Autodesk Inventor part; units mm, degrees
ref_plane "YZ Plane" through (0, 0, 0) normal (1, 0, 0) x (0, 1, 0)
ref_plane "XZ Plane" through (0, 0, 0) normal (0, 1, 0) x (-1, 0, 0)
ref_plane "XY Plane" through (0, 0, 0) normal (0, 0, 1) x (1, 0, 0)
sketch "Sketch1" plane through (0, 0, 0) normal (0, 1, 0) x (-1, 0, 0)
  circle A0 centre (0, 0) radius 100
  dimension "d0" = 200
extrude "Extrusion1" add sketch "Sketch1" along normal blind 40
sketch "Sketch2" plane through (0, 40, 0) normal (0, 1, 0) x (1, 0, 0)
  circle A0 centre (0, 0) radius 90
  dimension "d3" = 180
extrude "Extrusion2" add sketch "Sketch2" along normal blind 5
sketch "Sketch3" plane through (0, 45, 0) normal (0, 1, 0) x (1, 0, 0)
  point P0 (0, 0)
sketch "Sketch4" plane through (0, 45, 0) normal (0, 1, 0) x (1, 0, 0)
  point P0 (0, 0)
sketch "Sketch5" plane through (0, 45, 0) normal (0, 1, 0) x (1, 0, 0)
  line L0 (-5, -90) -> (5, -90)
  line L1 (5, -90) -> (5, 90)
  line L2 (5, 90) -> (-5, 90)
  line L3 (-5, 90) -> (-5, -90)
  line L4 (-5, -90) -> (5, 90) construction
  line L5 (5, -90) -> (-5, 90) construction
  point P0 (0, 0)
  dimension "d6" = 10
  dimension "d7" = 180
extrude "Extrusion3" cut sketch "Sketch5" against normal blind 5
sketch "Sketch6" plane through (0, 45, 0) normal (0, 1, 0) x (1, 0, 0)
  line L0 (-90, 5) -> (90, 5)
  line L1 (90, 5) -> (90, -5)
  line L2 (90, -5) -> (-90, -5)
  line L3 (-90, -5) -> (-90, 5)
  line L4 (-90, 5) -> (90, -5) construction
  line L5 (90, 5) -> (-90, -5) construction
  point P0 (0, 0)
  dimension "d10" = 180
  dimension "d11" = 10
extrude "Extrusion4" cut sketch "Sketch6" against normal blind 5
sketch "Sketch7" plane through (0, 40, 0) normal (0, 1, 0) x (1, 0, 0)
  point P0 (0, 0)
sketch "Sketch8" plane through (0, 40, 0) normal (0, 1, 0) x (1, 0, 0)
  circle A0 centre (0, 0) radius 50
  dimension "d14" = 100
extrude "Extrusion6" cut sketch "Sketch8" along normal blind 10
sketch "Sketch10" plane through (0, 40, 0) normal (0, 1, 0) x (1, 0, 0)
  circle A0 centre (0, 0) radius 40
  dimension "d20" = 80
extrude "Extrusion7" add sketch "Sketch10" along normal blind 5
sketch "Sketch11" plane through (0, 0, 0) normal (0, -1, 0) x (1, 0, 0)
  circle A0 centre (85, 0) radius 7.5
  point P0 (0, 0)
  dimension "d23" = 15
extrude "Extrusion8" add sketch "Sketch11" along normal blind 5
pattern_circular "Circular Pattern1" count 6 over 360 about axis through (0, 0, 0) along (0, 1, 0) of "Extrusion8", "Extrusion1", "Extrusion7"
fillet "Fillet1" radius 159.1625 4 edges at (63.6396, 45, 63.6396) (-63.6396, 45, 63.6396) (-63.6396, 45, -63.6396) (63.6396, 45, -63.6396)
sketch "Sketch12" plane through (0, 45, 0) normal (0, 1, 0) x (1, 0, 0)
  point P0 (0, 0)
sketch "Sketch13" plane through (0, 45, 0) normal (0, 1, 0) x (1, 0, 0)
  circle A0 centre (-18.2246, -20.9627) radius 5
  point P0 (0, 0)
  dimension "d30" = 10
extrude "Extrusion9" add sketch "Sketch13" along normal mid plane 3
properties part number "Simon"
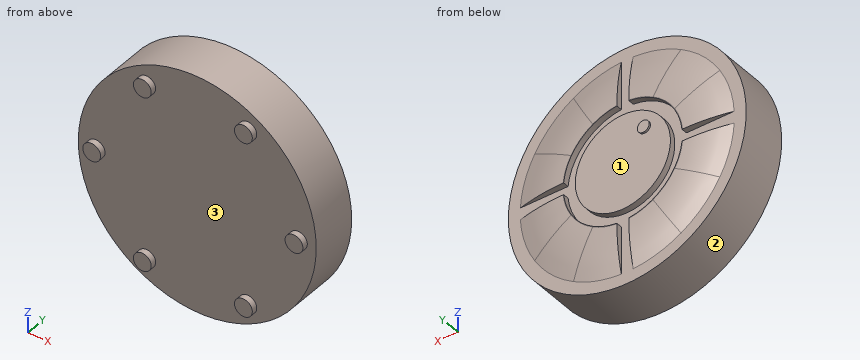
The listing builds one solid part. Answer for the finished solid, in the listing's coordinates (mm). Face numbers are marked on the shaded views. Give positions to 0.01 mm unless a question says otherwise; leave off trailing zeros. Write each loop counter-clockwise with the first axis right and the second up, starting at its lowest first coordinate (ties: lowest second). Pieces come first, ordered by that corner, then holes. Notation, with made-up numbers: M 35,89.25 L 40,89.25 A29 cw 40,119.25 Z; hole C 67,36 d3. An arc over 180 degrees is marked long. Write each question's results on one line, items separated by ' | '.
Q1. Section A-A, the plane z = 0 is taken. Write down the section's boundary in (x, y).
Output values:
outline: M -100,0 L -92.5,0 L -92.5,-5 L -77.5,-5 L -77.5,0 L 77.5,0 L 77.5,-5 L 92.5,-5 L 92.5,0 L 100,0 L 100,40 L 40,40 L 40,45 L -40,45 L -40,40 L -100,40 Z
Q2. Section B-B, the plane y = 18.5 is taken. Write down the section's boundary in (x, z), then the cut area to 3 significant figures.
Output values:
outline: C 0,0 d200 | area: 31,400 mm2
Q3. For a pull along X with two mould halves and no side action, classify the marked faces 1, 2 and 3 as released by +X, released by -X, zero draft, split by the parting line, or undercut.
Output values:
face 1: zero draft | face 2: split by the parting line | face 3: undercut
Q4. Consider L1, parallel to Y at x = 21, z = -38; L2, parallel to Z at x = -42, y = -1.5; L3, parallel to Y at x = -12.5, z = 23.5. Determine where each line is inside the solid, lowest interval first. Write a range as from..to.
Output values:
L1: 0..40 | L2: -81.1..-66.13, 66.13..81.1 | L3: 0..45
Q5. Flat-ended cylindrical pins translate along their axes: P1, Ø5, axis at x = 14.5, y = 38, coming from the -Z side; P2, Ø3, axis at y = 9, z = -39, coming from the -X side; P3, Ø13.5, axis at x = 18, z = 27, coming from the +Y side. Find the tip coordinate at first contact, or state that the pin passes through.
Output values:
P1: z = -99.28 | P2: x = -92.7 | P3: y = 45
